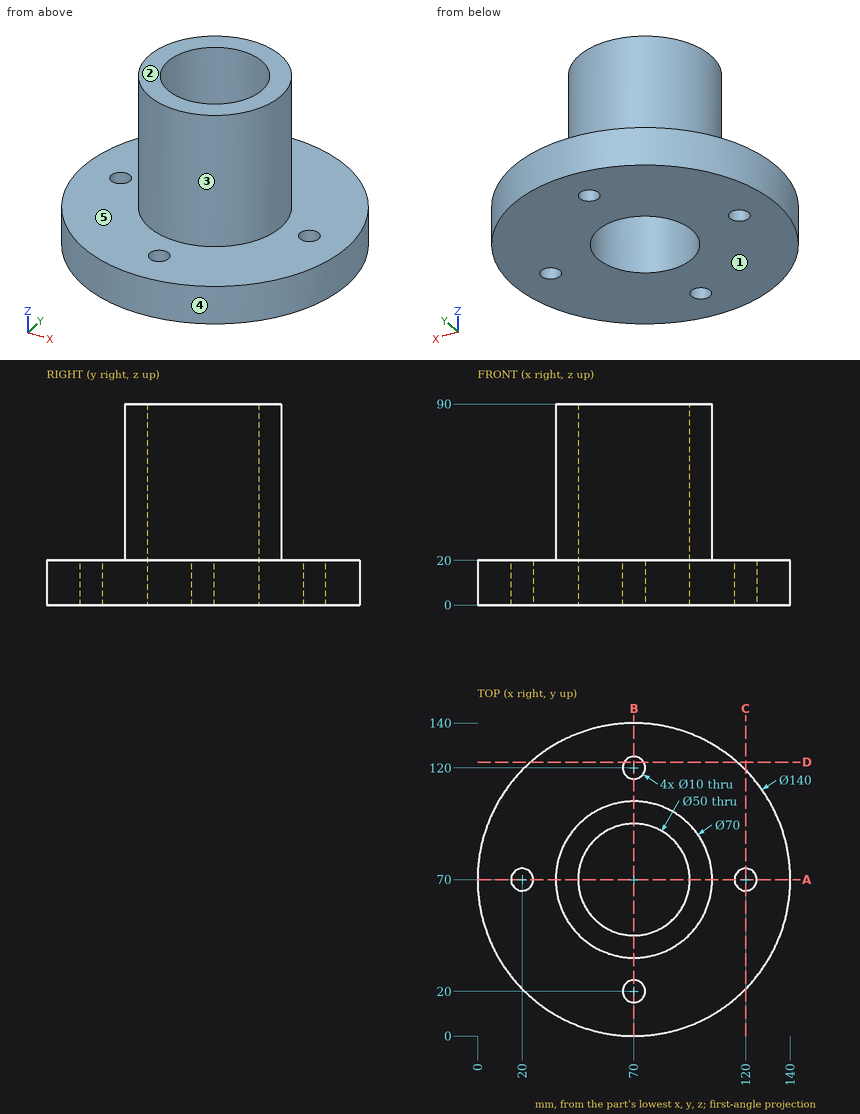
Input: dimensioned drawing with shaded views. Units: mm. Origin: part minimum x, y, z. A direction names the side the tool comes from. Give positions to 0.01 mm unless a question says otherwise; leave off trailing zeros. Loops run counter-clockwise (first coordinate to the right, second up) from the corner with the lowest first, then second, coordinate; pieces in that order, holes last. Notation, with made-up numbers: (-24, 40.5) - (11, 40.5) arc R19 ccw to (11, 61.5) - close; hole circle Ø9 at (54.5, 13.5). An arc over 180 degrees is marked (long way). Answer as CSV lines item,"result". Start each with the question number.
(1) Reachability of the marked faces 4 and 5 from +Z, -Z, +X, -X, +Y, -Y: full face, straight path, thin tool, end or side. Return the list, or none.
(2) Pin query (flat end, axial travel): P1, Ø11.5, axis at x = 20, y = 70, coming from the +Z side; P2, Ø2, axis at y = 38, z = 20.5, coming from the +X side; P3, Ø8, axis at y = 59, z = 63.5, coming from the +X side. Return the tip coordinate at first contact, or that it passes through.
(3) Ray query, line 1 along Y through (x, z) = (70, 8); line 2 along Y through (x, z) = (70, 67); line 3 along Z through (x, y) = (59.5, 25). Return the intervals inside material, ascending. Write a range as [from, to].
(4) Mould query, pull axis Z, two halves, no side actions, for the marked faces 1, 2 and 3. Classes: +Z half, -Z half, draft (parallel to the pull), parting line (faces both ways), or undercut.
(5) Section query A-A (y = 70). Output: boundary loops of the cut face in (x, z).
(6) Section query D-D (y = 122.5). Output: boundary loops of the cut face in (x, z).
(7) Section query C-C (x = 120). Output: boundary loops of the cut face in (y, z), and give its area (3 significant figures).
Worked answers:
1,face 4,"+Z, -Z"
1,face 5,"+Z"
2,P1,"stops at z = 20"
2,P2,"stops at x = 132.7"
2,P3,"stops at x = 104.29"
3,line 1,"y = [0, 15], [25, 45], [95, 115], [125, 140]"
3,line 2,"y = [35, 45], [95, 105]"
3,line 3,"z = [0, 20]"
4,face 1,"-Z half"
4,face 2,"+Z half"
4,face 3,"draft"
5,outline,"(0, 0) - (15, 0) - (15, 20) - (0, 20) - close; (25, 0) - (45, 0) - (45, 90) - (35, 90) - (35, 20) - (25, 20) - close; (95, 0) - (115, 0) - (115, 20) - (105, 20) - (105, 90) - (95, 90) - close; (125, 0) - (140, 0) - (140, 20) - (125, 20) - close"
6,outline,"(23.7, 0) - (65.67, 0) - (65.67, 20) - (23.7, 20) - close; (74.33, 0) - (116.3, 0) - (116.3, 20) - (74.33, 20) - close"
7,outline,"(21.01, 0) - (65, 0) - (65, 20) - (21.01, 20) - close; (75, 0) - (118.99, 0) - (118.99, 20) - (75, 20) - close"
7,area,"1,760 mm^2"
